Work out the finished part from the listing and answer in its coordinate system (mm). Coordinates: 2 decimals unless noted, no trailing zeros. Loops run counter-clockwise (first coordinate to the right, second up) from the corner with the lowest first, then second, coordinate; pieces in that order, holes last. Notation, with made-up numbers: (85, 85) -> (119, 85) arc R26 cw to (119, 123) -> close; hole circle Ø4 at (33.25, -21). An arc over 180 degrees is marked (long way). One line per question, with ' | ' between items.
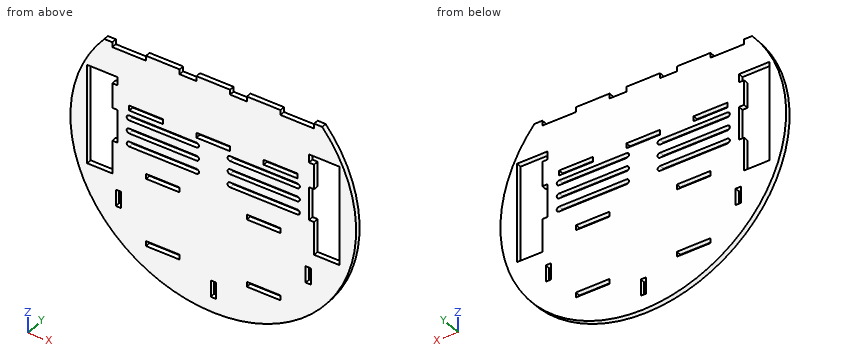
Autodesk Inventor part; units mm, degrees
ref_plane "YZ Plane" through (0, 0, 0) normal (1, 0, 0) x (0, 1, 0)
ref_plane "XZ Plane" through (0, 0, 0) normal (0, 1, 0) x (-1, 0, 0)
ref_plane "XY Plane" through (0, 0, 0) normal (0, 0, 1) x (1, 0, 0)
sketch "Sketch1" plane through (0, 0, 0) normal (0, 1, 0) x (-1, 0, 0)
  circle A0 centre (0, 0) radius 85
  line L0 (-64.8074, 55) -> (64.8074, 55)
  dimension "d0" = 170
  dimension "d1" = 55
extrude "Extrusion1" add sketch "Sketch1" along normal blind 3 contours A0 L0 picked at (-1.5877, 8.3779)
sketch "Sketch2" plane through (0, 3, 0) normal (0, 1, 0) x (1, 0, 0)
  line L0 (-75, 25) -> (-60, 25)
  line L1 (-60, 25) -> (-60, -35)
  line L2 (-60, -35) -> (-75, -35)
  line L3 (-75, -35) -> (-75, 25)
  line L4 (-75, -5) -> (-60, -5) construction
  point P0 (0, 0)
  dimension "d4" = 15
  dimension "d5" = 60
  dimension "d6" = 60
  dimension "d7" = 5
extrude "Extrusion2" cut sketch "Sketch2" against normal blind 3
sketch "Sketch3" plane through (0, 3, 0) normal (0, 1, 0) x (1, 0, 0)
  line L0 (-60, -35) -> (-60, 25)
  line L1 (-60, -15) -> (-57, -15)
  line L2 (-57, -15) -> (-57, 5)
  line L3 (-57, 5) -> (-60, 5)
  line L4 (-60, 5) -> (-60, -15)
  line L5 (-60, -35) -> (-57, -35)
  line L6 (-57, -35) -> (-57, -30)
  line L7 (-57, -30) -> (-60, -30)
  line L8 (-60, -30) -> (-60, -35)
  point P0 (0, 0)
  point P1 (-57, -5)
  point P2 (-60, -5)
  dimension "d10" = 3
  dimension "d11" = 20
  dimension "d12" = 3
  dimension "d13" = 5
  dimension "d14" = 15
extrude "Extrusion3" cut sketch "Sketch3" against normal blind 3
sketch "Sketch8" plane through (0, 3, 0) normal (0, 1, 0) x (1, 0, 0)
  line L0 (-10, -13) -> (-50, -13) construction
  line L1 (-10, -11.5) -> (-50, -11.5)
  line L2 (-50, -14.5) -> (-10, -14.5)
  arc A0 (-10, -14.5) -> (-10, -11.5) centre (-10, -13) ccw
  arc A1 (-50, -11.5) -> (-50, -14.5) centre (-50, -13) ccw
  line L3 (-10, -5) -> (-50, -5) construction
  line L4 (-10, -3.5) -> (-50, -3.5)
  line L5 (-50, -6.5) -> (-10, -6.5)
  arc A2 (-10, -6.5) -> (-10, -3.5) centre (-10, -5) ccw
  arc A3 (-50, -3.5) -> (-50, -6.5) centre (-50, -5) ccw
  line L6 (-10, 3) -> (-50, 3) construction
  line L7 (-10, 4.5) -> (-50, 4.5)
  line L8 (-50, 1.5) -> (-10, 1.5)
  arc A4 (-10, 1.5) -> (-10, 4.5) centre (-10, 3) ccw
  arc A5 (-50, 4.5) -> (-50, 1.5) centre (-50, 3) ccw
  point P0 (0, 0)
  point P1 (-30, -13)
  point P2 (-30, -5)
  point P3 (-30, 3)
  dimension "d54" = 3
  dimension "d55" = 3
  dimension "d56" = 3
  dimension "d57" = 5
  dimension "d58" = 5
  dimension "d59" = 5
  dimension "d60" = 40
  dimension "d61" = 30
extrude "Extrusion7" cut sketch "Sketch8" against normal blind 3
sketch "Sketch4" plane through (0, 3, 0) normal (0, 1, 0) x (1, 0, 0)
  line L0 (-60, -55) -> (-40, -55)
  line L1 (-40, -55) -> (-40, -52)
  line L2 (-40, -52) -> (-60, -52)
  line L3 (-60, -52) -> (-60, -55)
  line L4 (-64.8074, -55) -> (64.8074, -55)
  line L5 (-20, -55) -> (-10, -55)
  line L6 (-10, -55) -> (-10, -52)
  line L7 (-10, -52) -> (-20, -52)
  line L8 (-20, -52) -> (-20, -55)
  point P0 (0, 0)
  dimension "d17" = 20
  dimension "d18" = 3
  dimension "d19" = 10
  dimension "d20" = 3
  dimension "d21" = 10
  dimension "d22" = 20
extrude "Extrusion4" cut sketch "Sketch4" against normal blind 3
sketch "Sketch5" plane through (0, 0, 0) normal (0, -1, 0) x (1, 0, 0)
  line L0 (-50, 17.5) -> (-30, 17.5)
  line L1 (-30, 17.5) -> (-30, 20.5)
  line L2 (-30, 20.5) -> (-50, 20.5)
  line L3 (-50, 20.5) -> (-50, 17.5)
  line L4 (-10, 17.5) -> (10, 17.5)
  line L5 (10, 17.5) -> (10, 20.5)
  line L6 (10, 20.5) -> (-10, 20.5)
  line L7 (-10, 20.5) -> (-10, 17.5)
  line L8 (30, 17.5) -> (50, 17.5)
  line L9 (50, 17.5) -> (50, 20.5)
  line L10 (50, 20.5) -> (30, 20.5)
  line L11 (30, 20.5) -> (30, 17.5)
  point P0 (0, 0)
  dimension "d25" = 17.5
  dimension "d26" = 3
  dimension "d27" = 30
  dimension "d28" = 20
  dimension "d31" = 40
extrude "Extrusion5" cut sketch "Sketch5" against normal blind 3
sketch "Sketch6" plane through (0, 3, 0) normal (0, 1, 0) x (1, 0, 0)
  point P0 (0, 0)
sketch "Sketch7" plane through (0, 3, 0) normal (0, 1, 0) x (1, 0, 0)
  line L0 (55, 20) -> (-55, 20) construction
  line L1 (-55, 20) -> (-55, 58) construction
  line L2 (-55, 58) -> (55, 58) construction
  line L3 (55, 58) -> (55, 20) construction
  line L4 (40, 58) -> (20, 58)
  line L5 (20, 58) -> (20, 61)
  line L6 (20, 61) -> (40, 61)
  line L7 (40, 61) -> (40, 58)
  line L8 (-40, 58) -> (-20, 58)
  line L9 (-20, 58) -> (-20, 61)
  line L10 (-20, 61) -> (-40, 61)
  line L11 (-40, 61) -> (-40, 58)
  line L12 (40, 20) -> (20, 20)
  line L13 (20, 20) -> (20, 17)
  line L14 (20, 17) -> (40, 17)
  line L15 (40, 17) -> (40, 20)
  line L16 (-20, 20) -> (-40, 20)
  line L17 (-40, 20) -> (-40, 17)
  line L18 (-40, 17) -> (-20, 17)
  line L19 (-20, 17) -> (-20, 20)
  line L20 (55, 34) -> (58, 34)
  line L21 (58, 34) -> (58, 44)
  line L22 (58, 44) -> (55, 44)
  line L23 (55, 44) -> (55, 34)
  line L24 (-55, 34) -> (-58, 34)
  line L25 (-58, 34) -> (-58, 44)
  line L26 (-58, 44) -> (-55, 44)
  line L27 (-55, 44) -> (-55, 34)
  point P0 (0, 0)
  point P1 (0, 58)
  point P2 (58, 39)
  point P3 (55, 39)
  dimension "d38" = 110
  dimension "d39" = 38
  dimension "d40" = 20
  dimension "d41" = 20
  dimension "d42" = 3
  dimension "d43" = 20
  dimension "d44" = 3
  dimension "d45" = 20
  dimension "d46" = 40
  dimension "d47" = 3
  dimension "d50" = 3
  dimension "d51" = 10
  dimension "d52" = 3
  dimension "d53" = 10
extrude "Extrusion6" cut sketch "Sketch7" against normal blind 3
mirror "Mirror1" about plane through (0, 0, 0) normal (1, 0, 0) of "Extrusion2", "Extrusion3", "Extrusion4", "Extrusion7"
sketch "Sketch9" plane through (0, 3, 0) normal (0, 1, 0) x (1, 0, 0)
  line L0 (1.5, 66) -> (-1.5, 66)
  line L1 (-1.5, 66) -> (-1.5, 76)
  line L2 (-1.5, 76) -> (1.5, 76)
  line L3 (1.5, 76) -> (1.5, 66)
  line L4 (20, 61) -> (40, 61)
  point P0 (0, 0)
  point P1 (0, 66)
  dimension "d64" = 3
  dimension "d65" = 10
  dimension "d66" = 5
extrude "Extrusion8" cut sketch "Sketch9" against normal blind 3
properties part number "BasePlate"
1) Find section D-D (z = 1.5). Write down the section's boundary in (x, y).
Check values:
outline: (-84.99, 0) -> (-75, 0) -> (-75, 3) -> (-84.99, 3) -> close; (-57, 0) -> (57, 0) -> (57, 3) -> (-57, 3) -> close; (75, 0) -> (84.99, 0) -> (84.99, 3) -> (75, 3) -> close
2) Find section C-C (y = 2.1). State how many separate pieces and enclosed holes the cut face has, plus the area to 3 significant figures.
Check values:
separate pieces: 1 | enclosed holes: 18 | area: 16,600 mm^2
3) Flat-ended cylindrical pins translate along their axes: pin 1 (1.5 mm diameter, centred on x = 42, y = 2, fed in from -Z); pin 2 (1.5 mm diameter, centred on y = 1.5, z = 53.5, fed in from -X); pin 3 (1.5 mm diameter, centred on y = 2, z = 18.5, fed in from -X). Find the tip coordinate at first contact, or state that the pin passes through.
Check values:
pin 1: stops at z = -74.32 | pin 2: stops at x = -66.65 | pin 3: stops at x = -83.13
4) Find section B-B (x = 67). Write down the section's boundary in (y, z).
Check values:
outline: (0, -52.31) -> (3, -52.31) -> (3, -25) -> (0, -25) -> close; (0, 35) -> (3, 35) -> (3, 52.31) -> (0, 52.31) -> close
5) Find the intervals of material crossed by line 1 along Z through (x, y) = (0.5, 1.05); line 2 along X through (y, z) = (2.75, 11); line 3 along Z through (x, y) = (-26.5, 1.3), in increasing order.
Check values:
line 1: z = -85 to -76, -66 to 17.5, 20.5 to 55 | line 2: x = -84.29 to -75, -57 to 57, 75 to 84.29 | line 3: z = -80.76 to -61, -58 to -20, -17 to -4.5, -1.5 to 3.5, 6.5 to 11.5, 14.5 to 55
6) Find section A-A (z = -68). Write down the section's boundary in (x, y), plus the area to 3 significant figures.
Check values:
outline: (-51, 0) -> (-1.5, 0) -> (-1.5, 3) -> (-51, 3) -> close; (1.5, 0) -> (51, 0) -> (51, 3) -> (1.5, 3) -> close | area: 297 mm^2
